```python
from build123d import *

# Parameters (mm, degrees)
SKETCH1_W           = 740.5
SKETCH1_H           = 80
BOSS_EXTRUDE1_DEPTH = 10
SKETCH2_W           = 11
SKETCH2_H           = 3
CUT_EXTRUDE1_DEPTH  = 741.5
SKETCH3_W           = 2
SKETCH3_H           = 2
CUT_EXTRUDE2_DEPTH  = 741.5
CUT_EXTRUDE4_DEPTH  = 81


with BuildPart() as part:
    # Sketch1 → Boss-Extrude1 (new body)
    with BuildSketch(Plane(origin=(0, 0, 0), x_dir=(1, 0, 0), z_dir=(0, 1, 0))):
        Rectangle(SKETCH1_W, SKETCH1_H)
    extrude(amount=BOSS_EXTRUDE1_DEPTH)

    # Sketch2 → Cut-Extrude1 (cut, through all)
    with BuildSketch(Plane.ZY.offset(370.25)):
        with Locations((34.5, 8.5)):
            Rectangle(SKETCH2_W, SKETCH2_H)
    extrude(amount=-CUT_EXTRUDE1_DEPTH, mode=Mode.SUBTRACT)

    # Sketch3 → Cut-Extrude2 (cut, through all)
    with BuildSketch(Plane.ZY.offset(370.25)):
        with Locations((37, 6)):
            Rectangle(SKETCH3_W, SKETCH3_H)
    extrude(amount=-CUT_EXTRUDE2_DEPTH, mode=Mode.SUBTRACT)

    # Sketch4 → Cut-Extrude4 (cut, through all)
    with BuildSketch(Plane(origin=(0, 0, -40), x_dir=(-1, 0, 0), z_dir=(0, 0, -1))):
        Polygon((-370.25, 0), (-360.25, 10), (-370.25, 10), align=None)
        Polygon((370.25, 10), (370.25, 0), (360.25, 10), align=None)
    extrude(amount=-CUT_EXTRUDE4_DEPTH, mode=Mode.SUBTRACT)


solid = part.part
```
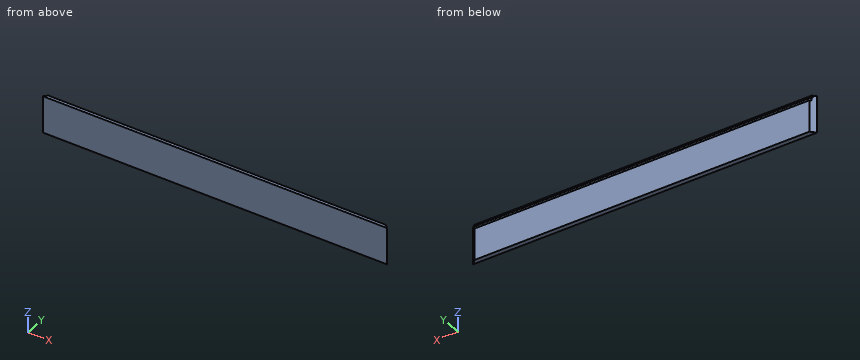
The listing builds one solid part. Answer for the finished solid, in the listing's coordinates (mm). Give positions to 0.01 mm unless a question says otherwise; leave off trailing zeros. Write each loop counter-clockwise with the first axis right and the second up, starting at its lowest first coordinate (ties: lowest second). Pieces come first, ordered by that corner, then holes. Notation, with made-up numbers: (5.5, 55) -> (53.5, 55) arc R19 ccw to (53.5, 87) -> close; hole circle Ø6 at (66, 64). An arc over 180 degrees is marked (long way). Use one line per item in the form item = value.
1) Section A-A on x = -13 is taken. Write down the section's boundary in (y, z), plus the area to 3 significant figures.
Result:
outline = (0, -40) -> (10, -40) -> (10, 29) -> (7, 29) -> (7, 36) -> (5, 36) -> (5, 38) -> (7, 38) -> (7, 40) -> (0, 40) -> close
area = 763 mm²
2) Straight lines are drawn through the part: probe 1 along Z at (x, y) = (78.5, 6.5); probe 2 along Z at (x, y) = (-102, 9); probe 3 along X at (y, z) = (6, -15). For each, find the intervals that lie inside material, in ascending order.
Result:
probe_1 = -40 to 36, 38 to 40
probe_2 = -40 to 29
probe_3 = -364.25 to 364.25
3) Each of these flat-tipped pins is pushed along its axis until it touches: P1, Ø3.5, axis at x = 160.5, y = 9, coming from the +Z side; P2, Ø1.5, axis at y = 2, z = 19.5, coming from the +X side; P3, Ø1.5, axis at y = 4, z = 15.5, coming from the -X side; P4, Ø10, axis at x = -103.5, z = 31, coming from the +Y side. Where does it stop, or does it pass through?
Result:
P1 = 29
P2 = 369
P3 = -367
P4 = 10
